```python
from build123d import *

# Parameters (mm, degrees)
F1_W     = 109.097563
F1_H     = 53.524394
F2_DEPTH = 10
F3_DEPTH = 20


with BuildPart() as f2:
    # F1 (on Top) → F2 (new body)
    with BuildSketch(Plane.XY):
        with Locations((5.012195, -4.353659)):
            Rectangle(F1_W, F1_H)
    extrude(amount=F2_DEPTH)

    # F0 (on Top) → F3 (cut)
    with BuildSketch(Plane.XY):
        with BuildLine():
            Line((-26.364613, 9.846089), (-43.052651, -21.557298))
            Line((-43.052651, -21.557298), (-43.142425, -22.709178))
            Line((-43.142425, -22.709178), (-34.816019, -22.603145))
            Line((-34.816019, -22.603145), (-28.477928, -10.9628))
            ThreePointArc((-28.477928, -10.9628), (-15.283365, -22.24516), (0, -14.010665))
            ThreePointArc((0, -14.010665), (13.880615, -22.568922), (26.360214, -12.072501))
            ThreePointArc((26.360214, -12.072501), (32.951882, -20.034667), (43.082863, -22.086348))
            ThreePointArc((43.082863, -22.086348), (53.397943, -12.183006), (50.914932, 1.899313))
            Line((50.914932, 1.899313), (43.082863, 1.899313))
            Line((43.082863, 1.899313), (46.387725, -7.834185))
            ThreePointArc((46.387725, -7.834185), (42.258111, -14.575967), (35.160247, -11.093775))
            Line((35.160247, -11.093775), (30.033628, 1.890382))
            Line((30.033628, 1.890382), (22.634767, 1.890382))
            ThreePointArc((22.634767, 1.890382), (18.111447, 3.978891), (13.189652, 4.752347))
            Line((13.189652, 4.752347), (13.189652, -2.555878))
            ThreePointArc((13.189652, -2.555878), (14.14297, -14.558516), (10.462902, -3.094257))
            Line((10.462902, -3.094257), (10.462902, 4.45175))
            ThreePointArc((10.462902, 4.45175), (9.026828, 4.192809), (7.681897, 3.626666))
            Line((7.681897, 3.626666), (-0.908288, 16.265618))
            Line((-0.908288, 16.265618), (-0.908288, -1.342427))
            ThreePointArc((-0.908288, -1.342427), (-5.880712, 2.929485), (-12.223111, 4.587256))
            Line((-12.223111, 4.587256), (-12.223111, -2.931808))
            ThreePointArc((-12.223111, -2.931808), (-13.936555, -14.910842), (-15.461971, -2.906415))
            Line((-15.461971, -2.906415), (-15.461971, 4.444678))
            ThreePointArc((-15.461971, 4.444678), (-18.558733, 3.847866), (-21.313343, 2.312209))
            Line((-21.313343, 2.312209), (-17.694002, 9.846089))
            Line((-17.694002, 9.846089), (-7.994306, 9.846089))
            Line((-7.994306, 9.846089), (-4.793087, 16.685043))
            Line((-4.793087, 16.685043), (-42.691354, 16.042456))
            Line((-42.691354, 16.042456), (-38.386457, 9.846089))
            Line((-38.386457, 9.846089), (-26.364613, 9.846089))
        make_face()
    extrude(amount=F3_DEPTH, mode=Mode.SUBTRACT)


solid = f2.part
```
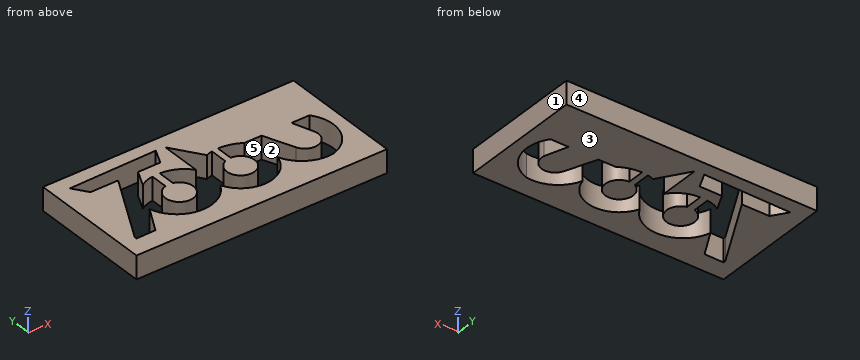
Here's how the part is built. I have some questions about the finished solid (model axes, mm). Face numbers are marked on the shaded views. A direction names the side the tool comes from. Round coordinates to 2 decimals unless told otherwise and drop trailing zeros. Order: outer loops, then holes, each group sorted by start corner. A loop starts at its lowest first (then second) coordinate and runs counter-clockwise, first axis right, second up. Notation, with made-up numbers: M 74.25,23.5 L 114.25,23.5 A27 ccw 114.25,55.5 Z; hole C 79,2.5 d11. An arc over 180 degrees is marked long. One line per question, with ' | ' between items.
1) I need wall thicknesses on line 1 along Y through (x, z) = (40.5, 5.75); line 2 along Y through (x, z) = (-8.5, 4.75); line 3 along Y through (x, z) = (9.5, 5.75). Which ranges of each line are inside material? Lowest first, please.
Working result:
line 1: -31.12 to -22.23, -14.81 to 22.41 | line 2: -31.12 to -21.44, -11.68 to -5.94, 3.99 to 9.85, 16.62 to 22.41 | line 3: -31.12 to -22.19, -13.58 to -3.64, 4.31 to 22.41
2) I want a section at D-D, the plane x = -11. Write out the boundary of the cut face in (y, z), then the cut area to 3 significant figures.
Working result:
outline: M -31.12,0 L -22.1,0 L -22.1,10 L -31.12,10 Z; M -14.18,0 L -3.43,0 L -3.43,10 L -14.18,10 Z; M 4.5,0 L 9.85,0 L 9.85,10 L 4.5,10 Z; M 16.58,0 L 22.41,0 L 22.41,10 L 16.58,10 Z | area: 309 mm²
3) For the marked faces 1 and 2, which set-ups out of +Z, -Z, +X, -X, +Y, -Y let a thin tool reach every point of the face, with its end or its side?
Working result:
face 1: +Z, -Z, +X, +Y, -Y | face 2: +Z, -Z
4) If we mould it in two halves opening along Y, with no side actions, what happens to the marked faces 3, 4 and 5? For each: +Y half, -Y half, draft (parallel to the pull), parting line (faces both ways), or undercut.
Working result:
face 3: draft | face 4: +Y half | face 5: undercut
5) I want a section at A-A, the plane x = 5. Write out the boundary of the cut face in (y, z).
Working result:
outline: M -31.12,0 L -20.17,0 L -20.17,10 L -31.12,10 Z; M 7.57,0 L 22.41,0 L 22.41,10 L 7.57,10 Z
6) I want a section at C-C, the plane x = 18. Write out the boundary of the cut face in (y, z), then the cut area to 3 significant figures.
Working result:
outline: M -31.12,0 L -21.62,0 L -21.62,10 L -31.12,10 Z; M -11.99,0 L -5.23,0 L -5.23,10 L -11.99,10 Z; M 4.01,0 L 22.41,0 L 22.41,10 L 4.01,10 Z | area: 346 mm²
7) I want a section at B-B, the plane y = -16. Write out the boundary of the cut face in (x, z).
Working result:
outline: M -49.54,0 L -40.1,0 L -40.1,10 L -49.54,10 Z; M -31.22,0 L -26.07,0 L -26.07,10 L -31.22,10 Z; M -1.22,0 L 1.02,0 L 1.02,10 L -1.22,10 Z; M 24.7,0 L 28.49,0 L 28.49,10 L 24.7,10 Z; M 51.53,0 L 59.56,0 L 59.56,10 L 51.53,10 Z
